Can you work these out from the model? Positions are in its coordinate system, mm. A direction names the side the tool comes from. Coordinates: 2 decimals unless noted, no trailing zeros. Order: outer loops, then holes, each group sorted by start corner. A loop starts at its lowest first (then second) coordinate and runs counter-clockwise, first axis right, second up. Notation, with made-up numbers: (68, 66.25) - (106, 66.25) arc R13 cw to (106, 86.25) - close; hole circle Ø11 at (27, 44.5). An arc over 180 degrees is marked (long way). Return JSON: item names as keys, results as strings. Group by question number.
1) If I drill on line 1 along Y through (x, z) = (-2.25, -7.75); line 2 along Y through (x, z) = (-6, -7); line 3 along X through (y, z) = (9.75, 1.75), over which ranges is the centre line in solid material (lowest first)?
2) Imagine slicing it at C-C (y = 7.25). Write out the boundary of the cut face in (x, z), and give its area (3 significant figures).
3) For pin 1 Ø2 at (x, y) = (-3.5, 10.5) entering from -Z; pin 2 Ø2 at (y, z) = (3, -6.5) entering from -X; pin 3 Ø1.5 at (x, y) = (-6.5, 2) entering from +Z, each with a flat end and sliding along its axis, tell me the tip position at first contact or that it passes through.
4) Imagine slicing it at A-A (z = 0). Write out the boundary of the cut face in (x, y) (1 decimal), and give its area (3 significant figures).
5) If we mould it in two halves opening along Y, with no side actions, what happens to faces 1 (the face through (0, 12.7, 0)), 2 (the face through (1.43, 4.31, -6.46)), 3 (the face through (0, 0, 0))? For each: pulls with the +Y half, pulls with the -Y half, needs draft (parallel to the pull), parting line crosses it, or undercut.
6) Imagine slicing it at B-B (x = 0). Write out the boundary of the cut face in (y, z) (1 decimal).
7) Imagine slicing it at D-D (y = 10.5). Write out the boundary of the cut face in (x, z), and give its area (3 significant figures).
8) Which directions (+Z, -Z, +X, -X, +Y, -Y) give clear straight access to the entire face, cutting with the end or side of a thin tool? Please do faces 4 (the face through (2, 7.62, 6.4)), 5 (the face through (1.22, 1.2, 9.32)).
```python
from build123d import *

# Parameters (mm, degrees)
FILLET1_R      = 0.79375
CHAMFER1_SIZE  = 0.79375
CHAMFER1_SIZE2 = 1.374815329


with BuildPart() as part:
    # Sketch1 → Revolve1 (revolve)
    with BuildSketch(Plane.XY):
        Polygon((0, 0), (-9.398, 0), (-9.398, 1.5875), (-6.477, 4.445), (-6.477, 7.62), (-9.398, 7.62), (-9.398, 12.7), (0, 12.7), align=None)
    revolve(axis=Axis((0, 0, 0), (0, 1, 0)))

    # Fillet1
    fillet1_edges = [part.edges().sort_by_distance(p)[0] for p in [
        (9.398, 0, 0),
    ]]
    fillet(fillet1_edges, radius=FILLET1_R)

    # Chamfer1
    chamfer1_edges = [part.edges().sort_by_distance(p)[0] for p in [
        (9.398, 12.7, 0),
    ]]
    chamfer1_side = [part.faces().sort_by_distance(p)[0] for p in [
        (0, 12.7, 0),
    ]]
    chamfer(chamfer1_edges, length=CHAMFER1_SIZE, length2=CHAMFER1_SIZE2, reference=chamfer1_side[0])


solid = part.part
```
Calculated:
{
 "1": {"line 1": "0 to 2.89, 7.62 to 12.7", "line 2": "0.29 to 1.76, 7.62 to 11.63", "line 3": "-9.23 to 9.23"},
 "2": {"outline": "circle Ø12.95 at (0, 0)", "area": "132 mm2"},
 "3": {"pin 1": "z = -9.06", "pin 2": "x = -6.49", "pin 3": "z = 7.34"},
 "4": {"outline": "(-9.4, 0.8) arc R0.8 ccw to (-8.6, 0) - (8.6, 0) arc R0.8 ccw to (9.4, 0.8) - (9.4, 1.6) - (6.5, 4.4) - (6.5, 7.6) - (9.4, 7.6) - (9.4, 11.3) - (8.6, 12.7) - (-8.6, 12.7) - (-9.4, 11.3) - (-9.4, 7.6) - (-6.5, 7.6) - (-6.5, 4.4) - (-9.4, 1.6) - close", "area": "210 mm2"},
 "5": {"face 1": "pulls with the +Y half", "face 2": "undercut", "face 3": "pulls with the -Y half"},
 "6": {"outline": "(0, -8.6) arc R0.8 ccw to (0.8, -9.4) - (1.6, -9.4) - (4.4, -6.5) - (7.6, -6.5) - (7.6, -9.4) - (11.3, -9.4) - (12.7, -8.6) - (12.7, 8.6) - (11.3, 9.4) - (7.6, 9.4) - (7.6, 6.5) - (4.4, 6.5) - (1.6, 9.4) - (0.8, 9.4) arc R0.8 ccw to (0, 8.6) - close"},
 "7": {"outline": "circle Ø18.8 at (0, 0)", "area": "277 mm2"},
 "8": {"face 4": "none", "face 5": "+Y, -Y"}
}
